Check sheet for the modelled part. Datum: model origin and axes. Units: mm. A direction names the side the tool comes from. Round coordinates to 2 decimals unless told otherwise and drop trailing zeros. Write each loop counter-clockwise with the first axis right and the second up, starting at its lowest first coordinate (ties: lowest second). Pieces come first, ordered by that corner, then holes. Notation, with made-up numbers: (54, 74.5) -> (105, 74.5) arc R31 cw to (105, 112.5) -> close; hole circle Ø1 at (55.25, 77). An arc over 180 degrees is marked (long way). Write item = value, one per line.
from build123d import *

# Parameters (mm, degrees)
EXTRUDE_1_DEPTH             = 10
HOLE_WIZARD_M41_D           = 3.3
HOLE_WIZARD_M41_DEPTH       = 11.5
HOLE_WIZARD_M41_CSINK_D     = 4.05
HOLE_WIZARD_M41_CSINK_ANGLE = 120
HOLE_WIZARD_M41_TIP         = 0.991420021
HOLE_WIZARD_M42_D           = 3.3
HOLE_WIZARD_M42_DEPTH       = 11.5
HOLE_WIZARD_M42_CSINK_D     = 4.05
HOLE_WIZARD_M42_CSINK_ANGLE = 120
HOLE_WIZARD_M42_TIP         = 0.991420021
HOLE_WIZARD_M43_D           = 3.3
HOLE_WIZARD_M43_DEPTH       = 6
HOLE_WIZARD_M43_CSINK_D     = 4.05
HOLE_WIZARD_M43_CSINK_ANGLE = 120
HOLE_WIZARD_M43_TIP         = 0.991420021


with BuildPart() as part:
    # Эскиз1 → Бобышка-Вытянуть1 (new body)
    with BuildSketch(Plane.XY):
        Polygon((0, 0), (0, 8), (-22, 30), (-22, 47), (19, 47), (19, 0), align=None)
    extrude(amount=EXTRUDE_1_DEPTH)

    # Отверстие обработанное метчиком M41
    with Locations(Plane(origin=(19, 0, 0), x_dir=(0, 0, -1), z_dir=(1, 0, 0))):
        with Locations((-5, 40), (-5, 15)):
            CounterSinkHole(HOLE_WIZARD_M41_D / 2, HOLE_WIZARD_M41_CSINK_D / 2, depth=HOLE_WIZARD_M41_DEPTH, counter_sink_angle=HOLE_WIZARD_M41_CSINK_ANGLE)
            with Locations((0, 0, -(HOLE_WIZARD_M41_DEPTH + HOLE_WIZARD_M41_TIP / 2))):  # 118° drill point
                Cone(0, HOLE_WIZARD_M41_D / 2, HOLE_WIZARD_M41_TIP, mode=Mode.SUBTRACT)

    # Отверстие обработанное метчиком M42
    with Locations(Plane.ZY.offset(22)):
        with Locations((5, 37)):
            CounterSinkHole(HOLE_WIZARD_M42_D / 2, HOLE_WIZARD_M42_CSINK_D / 2, depth=HOLE_WIZARD_M42_DEPTH, counter_sink_angle=HOLE_WIZARD_M42_CSINK_ANGLE)
            with Locations((0, 0, -(HOLE_WIZARD_M42_DEPTH + HOLE_WIZARD_M42_TIP / 2))):  # 118° drill point
                Cone(0, HOLE_WIZARD_M42_D / 2, HOLE_WIZARD_M42_TIP, mode=Mode.SUBTRACT)

    # Отверстие обработанное метчиком M43
    with Locations(Plane(origin=(0, 47, 0), x_dir=(-1, 0, 0), z_dir=(0, 1, 0))):
        with Locations((18, 5)):
            CounterSinkHole(HOLE_WIZARD_M43_D / 2, HOLE_WIZARD_M43_CSINK_D / 2, depth=HOLE_WIZARD_M43_DEPTH, counter_sink_angle=HOLE_WIZARD_M43_CSINK_ANGLE)
            with Locations((0, 0, -(HOLE_WIZARD_M43_DEPTH + HOLE_WIZARD_M43_TIP / 2))):  # 118° drill point
                Cone(0, HOLE_WIZARD_M43_D / 2, HOLE_WIZARD_M43_TIP, mode=Mode.SUBTRACT)


solid = part.part
(1) Sectioned sample at D-D on x = -3.5. Enter the section's corners in (y, z).
Worked answers:
outline = (11.5, 0) -> (47, 0) -> (47, 10) -> (11.5, 10) -> close
(2) Material ranges on L1, parallel to Y at x = 13.25, z = 5; L2, parallel to X at y = 42.65, z = 5; L3, parallel to Z at x = -18, y = 44, recorded low to high. Write a range as [from, to].
Worked answers:
L1 = [0, 13.35], [16.65, 38.35], [41.65, 47]
L2 = [-22, -19.65], [-16.35, 19]
L3 = [0, 3.35], [6.65, 10]
(3) Go/stop test with flat-tipped pins: P1, Ø2.5, axis at y = 2, z = 7, coming from the -X side; P2, Ø2, axis at y = 40, z = 5, coming from the +X side; P3, Ø1.5, axis at y = 8, z = 3.5, coming from the -X side. Record where each tip stops, or that it passes through.
Worked answers:
P1 = 0
P2 = 7.11
P3 = -0.75
(4) Release check for a two-part mould opening along Z. For faces 4 (the cylindrical face through (-16.063, 38.115, 6.216)), 5 (the flat face through (10, 0, 5)), 6 (the flat face through (3, 29, 0)) record: pulls with the +Z half, pulls with the -Z half, needs draft (parallel to the pull), parting line crosses it, or undercut.
Worked answers:
face_4 = undercut
face_5 = needs draft
face_6 = pulls with the -Z half
(5) Sectioned sample at C-C on y = 18.5. Enter the section's corners in (x, z), then the cut area to 3 significant figures.
Worked answers:
outline = (-10.5, 0) -> (19, 0) -> (19, 10) -> (-10.5, 10) -> close
area = 295 mm²
(6) Access from +Z, -Z, +X, -X, +Y, -Y to the whole of each face (thin tool, end or side, straight path). Record for faces 1 (the flat face through (0, 4, 5)), 2 (the conical face through (-9.7, 36.7, 5.1)), 3 (the cylindrical face through (13.06, 15.07, 3.35)).
Worked answers:
face_1 = +Z, -Z, -X, -Y
face_2 = -X
face_3 = +X
(7) Sectioned sample at A-A on x = 12.5. Enter the section's corners in (y, z), then the cut area to 3 significant figures.
Worked answers:
outline = (0, 0) -> (47, 0) -> (47, 10) -> (0, 10) -> close; hole circle Ø3.3 at (15, 5); hole circle Ø3.3 at (40, 5)
area = 453 mm²
(8) Sectioned sample at B-B on x = -12. Enter the section's corners in (y, z).
Worked answers:
outline = (20, 0) -> (47, 0) -> (47, 10) -> (20, 10) -> close; hole circle Ø3.3 at (37, 5)
